Input: dimensioned drawing with shaded views. Units: mm. Origin: part minimum x, y, z. A direction names the side the tool comes from. Give positions to 0.01 mm unless a question says otherwise; leave off trailing zeros. Loops run counter-clockwise (first coordinate to the right, second up) from the corner with the lowest first, then second, coordinate; pieces in that order, holes last. Notation, with made-up numbers: (41.5, 22.5) -> (86.5, 22.5) arc R27 ccw to (86.5, 59.5) -> close; hole circle Ø10 at (-13.75, -9). An arc over 180 degrees is marked (long way). One line per question, with ' | ' between items. Start each with the question number.
Item 1: Section D-D on x = 22.75. Return loops of the section in (y, z).
Item 2: Section A-A on y = 8.75. Return loops of the section in (x, z).
Item 3: Mould query, pull axis Y, two halves, no side actions, for the marked faces 1, 2 and 3. Classes: released by +Y, released by -Y, zero draft, split by the parting line, or undercut.
Item 4: Pin query (flat end, axial travel): P1, Ø10, axis at y = 8.87, z = 9.43, coming from the +X side; P2, Ø8, axis at x = 10, z = 16, coming from the -Y side; P3, Ø1.5, axis at x = 6.5, z = 12, coming from the +Y side; P4, Ø2, axis at x = 20, z = 10, coming from the -Y side. Return the tip coordinate at first contact, or that it passes through.
Item 5: Set-up query: the marked faces 4, 5 and 6. Return all of +Z, -Z, +X, -X, +Y, -Y with unobstructed straight access to the full face (end or side cutting, diameter ignored); none if empty.
Item 6: Material intervals for line 1 along Y through (x, z) = (24, 8.5) (1 decimal); line 2 along Z through (x, y) = (22.75, 3.75) (1 decimal); line 3 along Z through (x, y) = (7.75, 14.25) (1 decimal), sorted ascending. Write a range as [from, to].
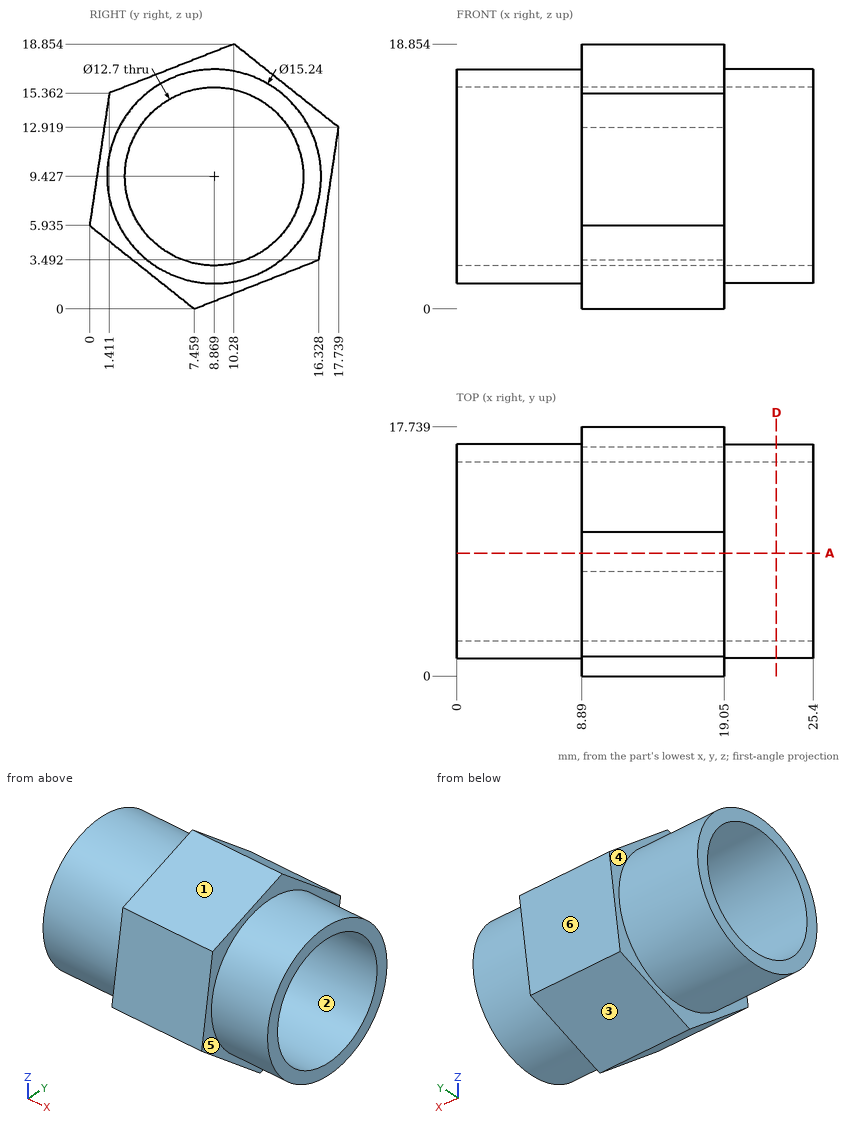
Result sheet:
1) outline: circle Ø15.24 at (8.87, 9.43); hole circle Ø12.7 at (8.87, 9.43)
2) outline: (0, 1.81) -> (8.89, 1.81) -> (8.89, 0.51) -> (19.05, 0.51) -> (19.05, 1.81) -> (25.4, 1.81) -> (25.4, 3.08) -> (0, 3.08) -> close; (0, 15.78) -> (25.4, 15.78) -> (25.4, 17.05) -> (19.05, 17.05) -> (19.05, 18.25) -> (8.89, 18.25) -> (8.89, 17.05) -> (0, 17.05) -> close
3) face 1: released by -Y | face 2: undercut | face 3: released by +Y
4) P1: passes through | P2: stops at y = 0.91 | P3: stops at y = 16.27 | P4: stops at y = 0.56
5) face 4: -X | face 5: +X | face 6: -Z, +X, -X, +Y
6) line 1: y = [1.3, 2.6], [15.2, 16.4] | line 2: z = [3.8, 5.7], [13.2, 15.1] | line 3: z = [4, 6.1], [12.8, 14.8]
